Autodesk Inventor part; units mm, degrees
ref_plane "YZ Plane" through (0, 0, 0) normal (1, 0, 0) x (0, 1, 0)
ref_plane "XZ Plane" through (0, 0, 0) normal (0, 1, 0) x (-1, 0, 0)
ref_plane "XY Plane" through (0, 0, 0) normal (0, 0, 1) x (1, 0, 0)
sketch "Sketch1" plane through (0, 0, 0) normal (0, 0, 1) x (1, 0, 0)
  line L0 (-36.7256, 32.4279) -> (36.0744, 32.4279)
  line L1 (36.0744, 32.4279) -> (36.0744, -37.5721)
  line L2 (36.0744, -37.5721) -> (-36.7256, -37.5721)
  line L3 (-36.7256, -37.5721) -> (-36.7256, 32.4279)
  point P0 (0, 0)
  dimension "d0" = 72.8
  dimension "d1" = 70
extrude "Extrusion1" add sketch "Sketch1" along normal blind 5
sketch "Sketch14" plane through (0, 0, 5) normal (0, 0, 1) x (1, 0, 0)
  line L0 (-33.0256, 28.7279) -> (32.3744, 28.7279)
  line L1 (32.3744, 28.7279) -> (32.3744, -4.0721)
  line L2 (32.3744, -4.0721) -> (-33.0256, -4.0721)
  line L3 (-33.0256, -4.0721) -> (-33.0256, 28.7279)
  line L4 (-36.7256, 32.4279) -> (-36.7256, -37.5721)
  line L5 (36.0744, -37.5721) -> (36.0744, 32.4279)
  line L6 (36.0744, 32.4279) -> (-36.7256, 32.4279)
  line L7 (-36.7256, -23.9721) -> (36.0744, -23.9721)
  point P0 (0, 0)
  dimension "d92" = 3.7
  dimension "d93" = 3.7
  dimension "d94" = 3.7
  dimension "d99" = 32.8
extrude "Extrusion13" add sketch "Sketch14" along normal blind 1 contours L0 L1 L2 L3
sketch "Sketch15" plane through (0, 0, 0) normal (0, 0, -1) x (-1, 0, 0)
  circle A0 centre (-33.5744, 29.9279) radius 1
  line L0 (36.7256, 32.4279) -> (-36.0744, 32.4279)
  line L1 (-36.0744, 32.4279) -> (-36.0744, -37.5721)
  line L2 (0.3256, 31.1231) -> (0.3256, 16.9299)
  circle A1 centre (34.2256, 29.9279) radius 1
  line L3 (-36.0744, -7.5721) -> (36.7256, -7.5721)
  line L4 (-36.0744, 12.4279) -> (-22.7568, 12.4279)
  circle A2 centre (-33.5744, -5.0721) radius 1
  circle A3 centre (34.2256, -5.0721) radius 1
  point P0 (0, 0)
  dimension "d100" = 2
  dimension "d101" = 2.5
  dimension "d102" = 2.5
  dimension "d103" = 40
  dimension "d104" = 20
hole "Hole2" at (33.5744, 29.9279, 0) at (-34.2256, 29.9279, 0) at (-34.2256, -5.0721, 0) at (33.5744, -5.0721, 0) direction (0, 0, 1) diameter 2 end through all countersink diameter 6 countersink angle 90
sketch "Sketch18" plane through (0, 0, 5) normal (0, 0, 1) x (1, 0, 0)
  line L0 (-36.7256, -37.5721) -> (-36.7256, -6.7304)
  line L1 (36.0744, -37.5721) -> (36.0744, 32.4279)
  line L2 (-36.7256, -7.9721) -> (36.0744, -7.9721)
  line L3 (36.0744, -7.9721) -> (36.0744, -23.8721)
  line L4 (36.0744, -23.8721) -> (-36.7256, -23.8721)
  line L5 (-36.7256, -23.8721) -> (-36.7256, -7.9721)
  line L6 (-33.0256, -4.0721) -> (32.3744, -4.0721)
  line L7 (-36.7256, -37.5721) -> (36.0744, -37.5721)
  point P0 (0, 0)
  dimension "d123" = 3.9
  dimension "d124" = 13.7
extrude "Extrusion16" add sketch "Sketch18" along normal blind 17 contours L0 L2 L1 L4
sketch "Sketch19" plane through (0, 0, 5) normal (0, 0, 1) x (1, 0, 0)
  line L0 (-36.7256, -37.5721) -> (36.0744, -37.5721)
  line L1 (-0.3256, -37.5721) -> (-0.3256, -23.8721)
  line L2 (-36.7256, -23.8721) -> (36.0744, -23.8721)
  circle A0 centre (-17.5256, -30.8221) radius 1
  circle A1 centre (16.8744, -30.8221) radius 1
  point P0 (0, 0)
  dimension "d127" = 2
  dimension "d128" = 2
  dimension "d129" = 6.75
  dimension "d130" = 6.75
  dimension "d131" = 17.2
  dimension "d132" = 17.2
extrude "Extrusion17" cut sketch "Sketch19" against normal through all
sketch "Sketch20" plane through (0, 0, 5) normal (0, 0, 1) x (1, 0, 0)
  line L0 (-6.3256, -27.8221) -> (5.6744, -27.8221)
  line L1 (5.6744, -27.8221) -> (5.6744, -33.8221)
  line L2 (5.6744, -33.8221) -> (-6.3256, -33.8221)
  line L3 (-6.3256, -33.8221) -> (-6.3256, -27.8221)
  line L4 (-36.7256, -37.5721) -> (36.0744, -37.5721)
  line L5 (-36.7256, -23.8721) -> (-36.7256, -37.5721)
  point P0 (0, 0)
  dimension "d135" = 12
  dimension "d136" = 6
  dimension "d137" = 3.75
  dimension "d138" = 30.4
extrude "Extrusion18" cut sketch "Sketch20" against normal through all
properties part number "Solonoid holder"
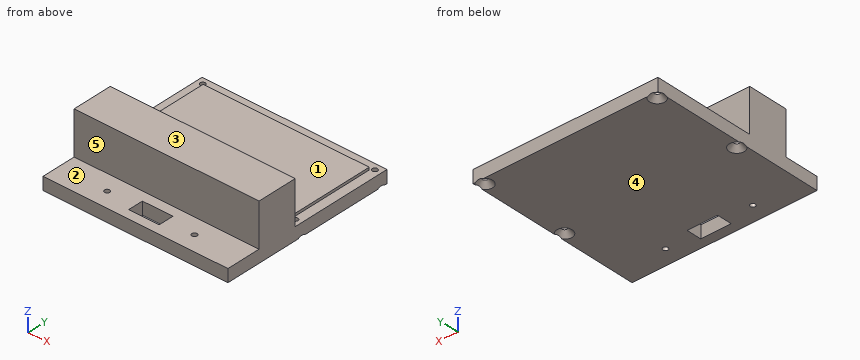
Geometry check sheet. Reference: the model listing, model coordinates, mm. Face numbers are marked on the shaded views. A direction names the side the tool comes from. Give positions to 0.01 mm unless a question says otherwise; leave off trailing zeros. Order: outer loops, then holes, each group sorted by start corner. A loop starts at its lowest first (then second) coordinate and runs counter-clockwise, first axis right, second up.
1. Sectioned sample at A-A (x = -1). Record the boundary of the cut face in (y, z).
Completed:
outline: (-37.57, 0) - (-33.82, 0) - (-33.82, 5) - (-37.57, 5) - close; (-27.82, 0) - (32.43, 0) - (32.43, 5) - (28.73, 5) - (28.73, 6) - (-4.07, 6) - (-4.07, 5) - (-7.97, 5) - (-7.97, 22) - (-23.87, 22) - (-23.87, 5) - (-27.82, 5) - close
2. Sectioned sample at C-C (x = 14). Record the boundary of the cut face in (y, z).
Completed:
outline: (-37.57, 0) - (32.43, 0) - (32.43, 5) - (28.73, 5) - (28.73, 6) - (-4.07, 6) - (-4.07, 5) - (-7.97, 5) - (-7.97, 22) - (-23.87, 22) - (-23.87, 5) - (-37.57, 5) - close
3. Depth check by flat-ended pin: pin 1 (6 mm diameter, centred on x = -23.5, y = 19, fed in from -Z); pin 2 (0.8 mm diameter, centred on y = 12, z = 5.5, fed in from -X); pin 3 (2.5 mm diameter, centred on x = 33.57, y = 29.93, fed in from +Z); pin 4 (8.5 mm diameter, centred on x = -13, z = 12.5, fed in from +Y). Enter the tip coordinate at first touch or a pass-through.
Completed:
pin 1: stops at z = 0
pin 2: stops at x = -33.03
pin 3: stops at z = 5
pin 4: stops at y = -7.97
4. Scan lines: line 1 (Y direction, x = 9, z = 5.25); line 2 (Y direction, x = -5, z = 3.75); line 3 (Y direction, x = -13.5, z = 19.25). Record each from-to range of solid material in increasing order.
Completed:
line 1: y = -23.87 to -7.97, -4.07 to 28.73
line 2: y = -37.57 to -33.82, -27.82 to 32.43
line 3: y = -23.87 to -7.97
5. Access from +Z, -Z, +X, -X, +Y, -Y to the whole of each face (thin tool, end or side, straight path). Record for the marked faces 1, 2 and 3.
Completed:
face 1: +Z, +X, -X, +Y
face 2: +Z, +X, -X, -Y
face 3: +Z, +X, -X, +Y, -Y
6. Sectioned sample at B-B (y = -1). Record the boundary of the cut face in (x, z).
Completed:
outline: (-36.73, 0) - (36.07, 0) - (36.07, 5) - (32.37, 5) - (32.37, 6) - (-33.03, 6) - (-33.03, 5) - (-36.73, 5) - close
7. Draft check along Y on the marked faces 4 and 5. Enter one of: pulls with the +Y half, pulls with the -Y half, needs draft (parallel to the pull), parting line crosses it, or undercut.
Completed:
face 4: needs draft
face 5: pulls with the -Y half
8. Sectioned sample at D-D (z = 15.5). Record the boundary of the cut face in (x, y), then the cut area to 3 significant figures.
Completed:
outline: (-36.73, -23.87) - (36.07, -23.87) - (36.07, -7.97) - (-36.73, -7.97) - close
area: 1,160 mm2
